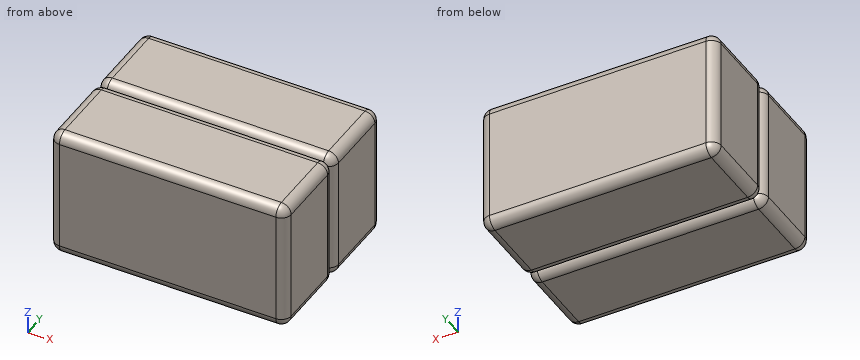
Solid Edge part; units mm, degrees
sketch "Sketch1" plane through (0, 0, 0) normal (0, 0, 1) x (1, 0, 0)
  line L0 (-36, 26) -> (36, 26)
  line L1 (36, 26) -> (36, 0)
  line L2 (36, 0) -> (-36, 0)
  line L3 (-36, 0) -> (-36, 26)
  dimension "D1" = 36
  dimension "D2" = 36
extrude "Protrusion1" add sketch "Sketch1" along normal mid plane 40
fillet "cell_rounds" radius 3 12 edges at (-36, 26, 0) (36, 26, 0) (36, 0, 0) (-36, 0, 0) (0, 0, 20) (36, 13, 20) (0, 26, 20) (-36, 13, 20) (0, 0, -20) (36, 13, -20) (0, 26, -20) (-36, 13, -20)
mirror "Mirror1" about plane through (0, 0, 0) normal (0, -1, 0) of "Protrusion1"
fillet "Round1" radius 3 12 edges at (-36, -26, 0) (-36, 0, 0) (36, 0, 0) (36, -26, 0) (36, -13, 20) (0, 0, 20) (-36, -13, 20) (0, -26, 20) (36, -13, -20) (0, 0, -20) (-36, -13, -20) (0, -26, -20)
properties material "ABS Plastic, medium impact"
Input: part model. Units: mm. Frame: model coordinates. Give positions to 0.01 mm unless a question says otherwise; leave off trailing zeros. Order: outer loops, then holes, each group sorted by start corner. A loop starts at its lowest first (then second) coordinate and runs counter-clockwise, first axis right, second up. Notation, with made-up numbers: (37, -4.5) - (43, -4.5) arc R14 cw to (43, 9.5) - close; hole circle Ø10 at (82, -9). An arc over 180 degrees is marked (long way). One line per item, written item: value.
1. Pin query (flat end, axial travel): pin 1 Ø6 at (y, z) = (1.5, -13) entering from -X; pin 2 Ø5 at (y, z) = (0, 3.5) entering from +X. Return the tip coordinate at first contact, or that it passes through.
Determined:
pin 1: x = -36
pin 2: x = 35.96
2. Cut plane A-A, the plane y = -2. Output: boundary loops of the cut face in (x, z).
Determined:
outline: (-35.83, -17) arc R2.83 ccw to (-33, -19.83) - (33, -19.83) arc R2.83 ccw to (35.83, -17) - (35.83, 17) arc R2.83 ccw to (33, 19.83) - (-33, 19.83) arc R2.83 ccw to (-35.83, 17) - close
3. Line query: probe 1 along Z at (x, y) = (27.5, -1); probe 2 along Z at (x, y) = (-18, 2); probe 3 along X at (y, z) = (2.5, -8). Output: solid intervals per line, ascending.
Determined:
probe 1: -19.24 to 19.24
probe 2: -19.83 to 19.83
probe 3: -35.96 to 35.96
